Check sheet for the drawn part. Datum: minimum x, y, z corner. Units: mm. A direction names the side the tool comes from. Coordinates: 2 decimals unless noted, no trailing zeros. Write each loop counter-clockwise with the first axis right and the second up, starting at its lowest first coordinate (ties: lowest second). Pieces come first, ordered by that corner, then holes. Notation, with made-up numbers: (-17, -24) -> (-1, -24) arc R12 ccw to (-1, -14) -> close; hole circle Ø10 at (49, 10). An arc over 180 degrees is marked (long way). One line per question, with ' | ' between items.
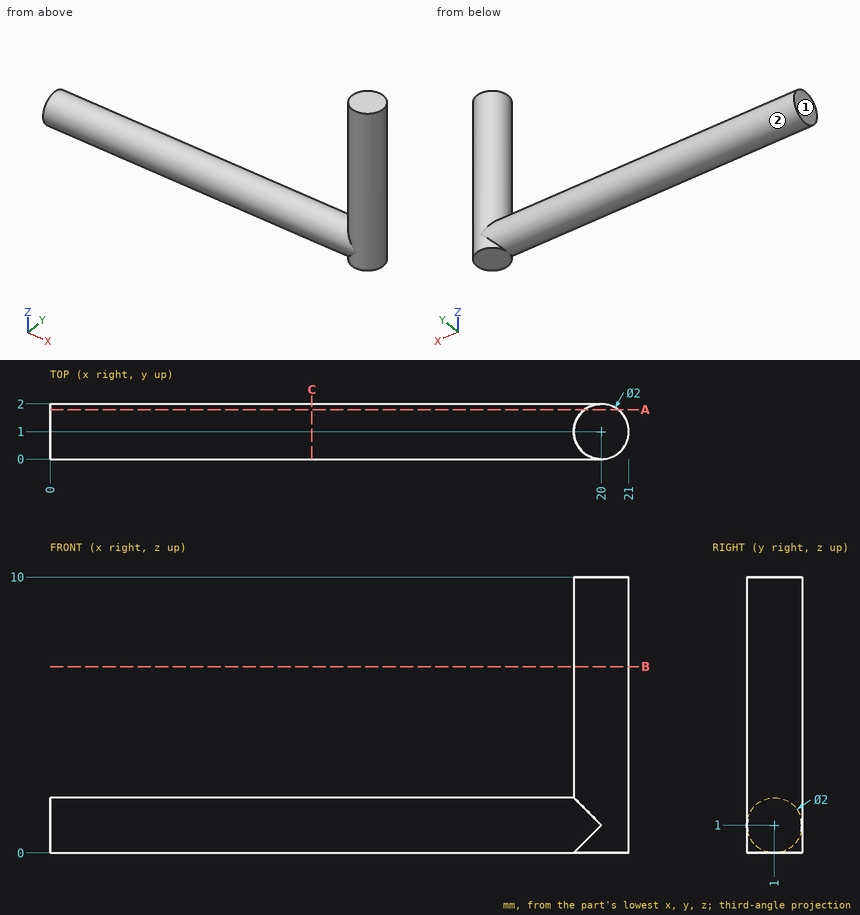
1. Cross-section at B-B on z = 6.75. Record the boundary of the cut face in (x, y), and give its area (3 significant figures).
Worked answers:
outline: circle Ø2 at (20, 1) | area: 3.14 mm²
2. Cross-section at C-C on x = 9.5. Record the boundary of the cut face in (y, z).
Worked answers:
outline: circle Ø2 at (1, 1)
3. Tool access check on the marked faces 1 and 2. Record the directions out of +Z, -Z, +X, -X, +Y, -Y that give a thin tool (end or side, any length) a straight path to the whole face; none if there is none.
Worked answers:
face 1: +Z, -Z, -X, +Y, -Y | face 2: -X
4. Cross-section at A-A on y = 1.8. Record the boundary of the cut face in (x, z).
Worked answers:
outline: (0, 0.4) -> (19.4, 0.4) -> (19.4, 0) -> (20.6, 0) -> (20.6, 10) -> (19.4, 10) -> (19.4, 1.6) -> (0, 1.6) -> close
5. Material ranges on line 1 (X direction, y = 0.9, z = 3.75); line 2 (X direction, y = 1.75, z = 2); line 3 (Z direction, x = 12.75, y = 1.05), recorded low to high. Write a range as from..to.
Worked answers:
line 1: 19.01..20.99 | line 2: 19.34..20.66 | line 3: 0..2
